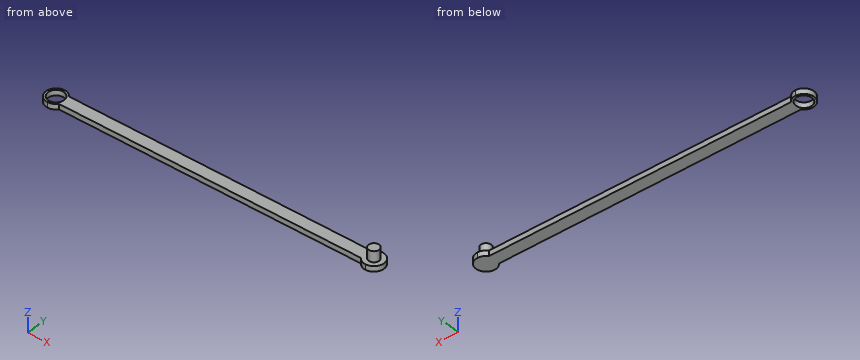
```python
from build123d import *

# Parameters (mm, degrees)
SKETCH1_R           = 1.5
BOSS_EXTRUDE1_DEPTH = 1
SKETCH38_R          = 0.975
BOSS_EXTRUDE2_DEPTH = 2


with BuildPart() as part:
    # Sketch1 → Boss-Extrude1 (new body)
    with BuildSketch(Plane.XY):
        with BuildLine():
            Line((1.497200651, 1.14350772), (58.502799349, 1.14350772))
            ThreePointArc((58.502799349, 1.14350772), (59.164858436, 1.688714974), (60, 1.883937285))
            ThreePointArc((60, 1.883937285), (61.883937285, 0), (60, -1.883937285))
            ThreePointArc((60, -1.883937285), (59.164858436, -1.688714974), (58.502799349, -1.14350772))
            Line((58.502799349, -1.14350772), (1.497200651, -1.14350772))
            ThreePointArc((1.497200651, -1.14350772), (0.835141564, -1.688714974), (0, -1.883937285))
            ThreePointArc((0, -1.883937285), (-1.883937285, 0), (0, 1.883937285))
            ThreePointArc((0, 1.883937285), (0.835141564, 1.688714974), (1.497200651, 1.14350772))
        make_face()
        Circle(SKETCH1_R, mode=Mode.SUBTRACT)
    extrude(amount=BOSS_EXTRUDE1_DEPTH)

    # Sketch38 → Boss-Extrude2 (add)
    with BuildSketch(Plane.XY.offset(1)):
        with Locations(Location((60, 0, 0), (0, 0, 180))):
            Circle(SKETCH38_R)
    extrude(amount=BOSS_EXTRUDE2_DEPTH)


solid = part.part
```
For this review, take the finished solid that the model builds, in its own axes (mm). Coordinates: 2 decimals unless noted, no trailing zeros. Write each loop counter-clockwise with the first axis right and the second up, starting at its lowest first coordinate (ties: lowest second). Pieces come first, ordered by that corner, then holes. Notation, with made-up numbers: (-18, 8.5) -> (1, 8.5) arc R11 ccw to (1, 17.5) -> close; hole circle Ø7 at (35.25, -40). An arc over 180 degrees is marked (long way). Put each result on its own line as item: value.
Q1. Wall thickness on L1, parallel to Y at x = 0, z = 0.25; L2, parallel to Z at x = 39, y = -0.5; L3, parallel to X at y = 1, z = 0.85: over which ranges is each line inside the solid? List them lowest first.
From the geometry:
L1: y = -1.88 to -1.5, 1.5 to 1.88
L2: z = 0 to 1
L3: x = -1.6 to -1.12, 1.12 to 61.6
Q2. Take a section at A-A, the plane y = 0. State the section outline as (x, z) points (3 decimals), then the cut area to 3 significant figures.
From the geometry:
outline: (-1.884, 0) -> (-1.5, 0) -> (-1.5, 1) -> (-1.884, 1) -> close; (1.5, 0) -> (61.884, 0) -> (61.884, 1) -> (60.975, 1) -> (60.975, 3) -> (59.025, 3) -> (59.025, 1) -> (1.5, 1) -> close
area: 64.7 mm2
Q3. Clearance check with flat-ended pins moving along their axes: pin 1 Ø0.5 at (x, z) = (29, 0.5) entering from -Y; pin 2 Ø0.5 at (x, z) = (37, 0.5) entering from +Y; pin 3 Ø1.5 at (x, y) = (24, 1) entering from +Z. State where each tip first meets the part, or that it passes through.
From the geometry:
pin 1: stops at y = -1.14
pin 2: stops at y = 1.14
pin 3: stops at z = 1
Q4. Take a section at B-B, the plane x = 56. State the section outline as (y, z) points.
From the geometry:
outline: (-1.14, 0) -> (1.14, 0) -> (1.14, 1) -> (-1.14, 1) -> close
Q5. Take a section at C-C, the plane z = 2.4. State the section outline as (x, y) points (3 decimals).
From the geometry:
outline: circle Ø1.95 at (60, 0)
